Geometry: final body of the model. Coordinates: model frame, mm. Coordinates: 2 decimals unless noted, no trailing zeros. Loops run counter-clockwise (first coordinate to the right, second up) from the corner with the lowest first, then second, coordinate; pieces in that order, holes last. Notation, with made-up numbers: (48, -17.5) - (75, -17.5) arc R9 cw to (75, -6.5) - close; hole circle Ø11 at (-14.75, 49). An arc over 180 degrees is marked (long way). Write each question's results on one line, items separated by ' | '. Start each with the question number.
Autodesk Inventor part; units mm, degrees
ref_plane "YZ Plane" through (0, 0, 0) normal (1, 0, 0) x (0, 1, 0)
ref_plane "XZ Plane" through (0, 0, 0) normal (0, 1, 0) x (-1, 0, 0)
ref_plane "XY Plane" through (0, 0, 0) normal (0, 0, 1) x (1, 0, 0)
sketch "Sketch1" plane through (0, 0, 0) normal (0, 1, 0) x (-1, 0, 0)
  line L0 (0, 0) -> (527.05, 0) construction
  line L1 (527.05, 0) -> (527.05, 787.4) construction
  line L2 (527.05, 787.4) -> (0, 787.4) construction
  line L3 (0, 787.4) -> (0, 0) construction
  line L4 (0, 787.4) -> (527.05, 0)
  line L5 (527.05, 0) -> (527.05, 50.8)
  line L6 (527.05, 0) -> (577.85, 0) construction
  line L7 (0, 787.4) -> (0, 838.2)
  line L8 (0, 787.4) -> (50.8, 787.4) construction
  line L9 (0, 838.2) -> (527.05, 50.8)
  dimension "d0" = 527.05
  dimension "d1" = 787.4
  dimension "d2" = 50.8
  dimension "d3" = 90
  dimension "d4" = 50.8
  dimension "d5" = 90
extrude "Extrusion1" add sketch "Sketch1" along normal blind 3.175
sketch "Sketch6" plane through (-527.05, 0, 0) normal (-1, 0, 0) x (0, 0, 1)
  line L0 (50.8, 0) -> (0, 0)
  line L1 (50.8, 0) -> (50.8, 3.175)
  line L2 (0, 3.175) -> (50.8, 3.175)
  line L3 (0, 0) -> (0, 3.175)
  line L4 (50.8, 0) -> (25.4, -25.4)
  line L5 (50.8, 0) -> (86.721, 0) construction
  line L6 (25.4, -25.4) -> (0, 0)
  dimension "d33" = 135
extrude "Extrusion4" add sketch "Sketch6" against normal blind 3.175
sketch "Sketch8" plane through (0, 3.175, 0) normal (0, 1, 0) x (1, 0, 0)
  line L0 (-527.05, 0) -> (-527.05, -50.8)
  line L1 (-527.05, -50.8) -> (0, -838.2)
  line L2 (0, -838.2) -> (0, -787.4)
  line L3 (0, -787.4) -> (-523.875, -4.7434)
  line L4 (-523.875, 0) -> (-523.875, -4.7434)
  line L5 (-527.05, 0) -> (-523.875, 0)
  line L6 (0, -838.2) -> (0, -812.8)
  line L7 (0, -787.4) -> (0, -838.2)
  line L8 (0, -812.8) -> (-17.0016, -812.8)
  line L9 (-17.0016, -812.8) -> (0, -838.2)
  line L10 (0, -838.2) -> (-527.05, -50.8)
  point P0 (0, 0)
extrude "Extrusion6" cut sketch "Sketch8" against normal blind 3.175 contours L8 L2 L1
sketch "Sketch9" plane through (-527.05, 0, 50.8) normal (-1, 0, 0) x (0, 0, 1)
  line L0 (0, 0) -> (0, 3.175)
  line L1 (-50.8, 3.175) -> (0, 3.175)
  line L2 (-50.8, 0) -> (-50.8, 3.175)
  line L3 (-50.8, 0) -> (-25.4, -25.4)
  line L4 (-25.4, -25.4) -> (0, 0)
  point P0 (-23.1549, -9.6846)
  dimension "d40" = 12.7
  dimension "d41" = 9.525
hole "Hole3" at (-527.05, -9.6846, 27.6451) direction (1, 0, 0) diameter 6.35 end through all
sketch "Sketch10" plane through (0, 3.175, 0) normal (0, 1, 0) x (1, 0, 0)
  line L0 (-17.0016, -812.8) -> (0, -812.8)
  line L1 (0, -812.8) -> (0, -787.4)
  line L2 (0, -787.4) -> (-523.875, -4.7434)
  line L3 (-523.875, 0) -> (-523.875, -4.7434)
  line L4 (-527.05, 0) -> (-523.875, 0)
  line L5 (-527.05, 0) -> (-527.05, -50.8)
  line L6 (-527.05, -50.8) -> (-17.0016, -812.8)
  point P0 (0, 0)
  point P1 (-12.7, -787.4)
  dimension "d52" = 12.7
  dimension "d53" = 25.4
hole "Hole4" at (-12.7, 3.175, 787.4) direction (0, -1, 0) diameter 6.35 end through all
properties part number "cross brace"
1) Section query A-A on z = 446. Output: boundary loops of the cut face in (x, y) (3 decimals), and give its area (3 significant figures).
2) Section query B-B on x = -185. Output: boundary loops of the cut face in (y, z) (3 decimals).
3) Material intervals for line 1 (Z direction, x = -12.7, y = 1.4) (1 decimal), sorted ascending. Write a range as [from, to].
4) Pin query (flat end, axial travel): pin 1 Ø2 at (x, y) = (-151.5, 0) entering from +Z. Return the tip coordinate at first contact, or that it passes through.
Returned:
1) outline: (-262.521, 0) - (-228.518, 0) - (-228.518, 3.175) - (-262.521, 3.175) - close | area: 108 mm²
2) outline: (0, 511.014) - (3.175, 511.014) - (3.175, 561.814) - (0, 561.814) - close
3) line 1: z = [768.4, 784.2], [790.6, 812.8]
4) pin 1: stops at z = 613.36
